Verification items for this drawing (mm, ordinates from the low corner). Give positions to 0.01 mm unless a question says otherwise; leave off trailing zeros. Loops run counter-clockwise (first coordinate to the right, second up) from the corner with the lowest first, then second, coordinate; pieces in that order, holes last. Notation, with made-up numbers: (85.5, 51) - (136.5, 51) arc R30 ccw to (136.5, 89) - close; hole circle Ø9 at (13.25, -26.5). An arc over 180 degrees is marked (long way). One line per question, with ' | ' between items. Start each with the question number.
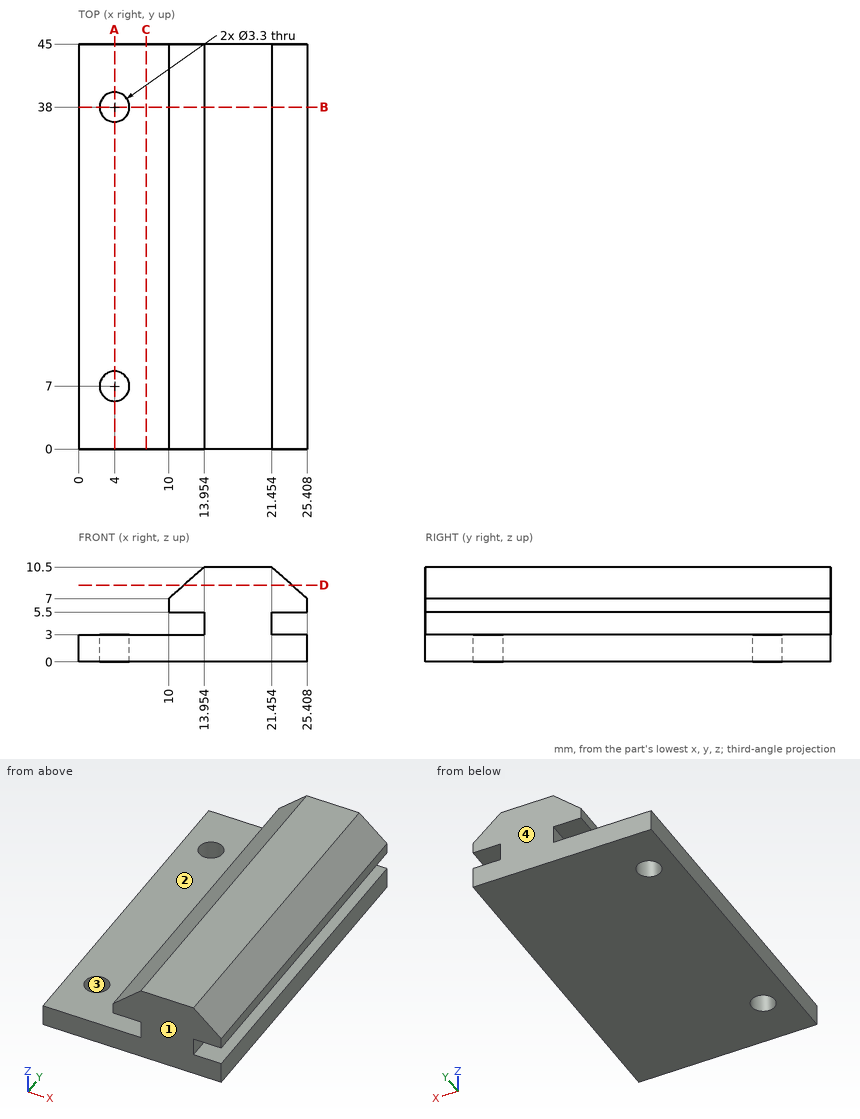
(1) Mould release check, pull along Y, two halves, no side actions. Record for the marked faces 1, 2, 3 and 4: pulls with the +Y half, pulls with the -Y half, needs draft (parallel to the pull), parting line crosses it, or undercut.
(2) Depth check by flat-ended pin: pin 1 Ø1.6 at (y, z) = (16, 6.5) entering from -X; pin 2 Ø3 at (x, y) = (24, 17.5) entering from +Z (1 decimal); pin 3 Ø2 at (x, y) = (4, 7) entering from -Z. Enter the tip coordinate at first touch or a pass-through.
(3) Material ranges on line 1 (Y direction, x = 4, z = 1.75); line 2 (X direction, y = 38, z = 1.25); line 3 (Z direction, x = 9, y = 32.5), recorded low to high.
(4) Section check D-D, the plane z = 8.5. Record the boundary of the cut face in (x, y) (1 decimal).
(5) Section check C-C, the plane x = 7.5. Record the boundary of the cut face in (y, z), and give its area (3 significant figures).
(6) Section check A-A, the plane x = 4. Record the boundary of the cut face in (y, z), and give its area (3 significant figures).
(7) Section check B-B, the plane y = 38. Record the boundary of the cut face in (x, z).
Numbers:
1) face 1: pulls with the -Y half | face 2: needs draft | face 3: undercut | face 4: pulls with the +Y half
2) pin 1: x = 10 | pin 2: z = 9.6 | pin 3: through
3) line 1: 0 to 5.35, 8.65 to 36.35, 39.65 to 45 | line 2: 0 to 2.35, 5.65 to 25.41 | line 3: 0 to 3
4) outline: (11.7, 0) - (23.7, 0) - (23.7, 45) - (11.7, 45) - close
5) outline: (0, 0) - (45, 0) - (45, 3) - (0, 3) - close | area: 135 mm^2
6) outline: (0, 0) - (5.35, 0) - (5.35, 3) - (0, 3) - close; (8.65, 0) - (36.35, 0) - (36.35, 3) - (8.65, 3) - close; (39.65, 0) - (45, 0) - (45, 3) - (39.65, 3) - close | area: 115 mm^2
7) outline: (0, 0) - (2.35, 0) - (2.35, 3) - (0, 3) - close; (5.65, 0) - (25.41, 0) - (25.41, 3) - (21.45, 3) - (21.45, 5.5) - (25.41, 5.5) - (25.41, 7) - (21.45, 10.5) - (13.95, 10.5) - (10, 7) - (10, 5.5) - (13.95, 5.5) - (13.95, 3) - (5.65, 3) - close
